```python
from build123d import *

# Parameters (mm, degrees)
SKETCH1_W                                            = 130
SKETCH1_H                                            = 10
BOSS_EXTRUDE1_DEPTH                                  = 10
CBORE_FOR_M3_HEXAGON_SOCKET_HEAD_CAP_SCR_D           = 3.2
CBORE_FOR_M3_HEXAGON_SOCKET_HEAD_CAP_SCR_CBORE_D     = 6
CBORE_FOR_M3_HEXAGON_SOCKET_HEAD_CAP_SCR_CBORE_DEPTH = 3.4
BOSS_EXTRUDE2_DEPTH                                  = 130


with BuildPart() as part:
    # Sketch1 → Boss-Extrude1 (new body)
    with BuildSketch(Plane.XY):
        with Locations((0, 5)):
            Rectangle(SKETCH1_W, SKETCH1_H)
    extrude(amount=BOSS_EXTRUDE1_DEPTH)

    # CBORE for M3 Hexagon socket head cap screws1 (through all)
    with Locations(Plane.XY.offset(10)):
        with Locations((-60, 5), (0, 5), (60, 5)):
            CounterBoreHole(CBORE_FOR_M3_HEXAGON_SOCKET_HEAD_CAP_SCR_D / 2, CBORE_FOR_M3_HEXAGON_SOCKET_HEAD_CAP_SCR_CBORE_D / 2, CBORE_FOR_M3_HEXAGON_SOCKET_HEAD_CAP_SCR_CBORE_DEPTH)

    # Sketch4 → Boss-Extrude2 (add)
    with BuildSketch(Plane.ZY.offset(65)):
        Polygon((10, 10), (0, 10), (0, 20), align=None)
    extrude(amount=-BOSS_EXTRUDE2_DEPTH)


solid = part.part
```
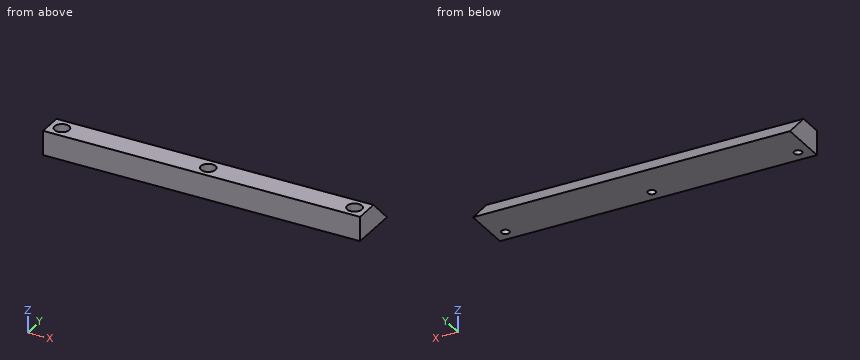
For this review, take the finished solid that the model builds, in its own axes (mm). Round coordinates to 2 decimals unless told otherwise and drop trailing zeros. Loops run counter-clockwise (first coordinate to the right, second up) from the corner with the lowest first, then second, coordinate; pieces in that order, holes last.
Q1. Add section D-D on y = 14.25. Write out the cut boundary in (x, z).
Result sheet:
outline: (-65, 0) - (65, 0) - (65, 5.75) - (-65, 5.75) - close
Q2. Add section A-A on y = 5. Write out the cut boundary in (x, z), plus the area to 3 significant figures.
Result sheet:
outline: (-65, 0) - (-61.6, 0) - (-61.6, 6.6) - (-63, 6.6) - (-63, 10) - (-65, 10) - close; (-58.4, 0) - (-1.6, 0) - (-1.6, 6.6) - (-3, 6.6) - (-3, 10) - (-57, 10) - (-57, 6.6) - (-58.4, 6.6) - close; (1.6, 0) - (58.4, 0) - (58.4, 6.6) - (57, 6.6) - (57, 10) - (3, 10) - (3, 6.6) - (1.6, 6.6) - close; (61.6, 0) - (65, 0) - (65, 10) - (63, 10) - (63, 6.6) - (61.6, 6.6) - close
area: 1,180 mm2
Q3. Insertion check: pin 1 Ø3.5 at (x, y) = (-60, 5) entering from +Z; pin 2 Ø3 at (x, y) = (0, 5) entering from +Z; pin 3 Ø1.5 at (x, y) = (48, 18) entering from +Z. Each pin has a flat end and moves straight along its axis. Give the tip position at first contact, or say it passes through.
Result sheet:
pin 1: stops at z = 6.6
pin 2: passes through
pin 3: stops at z = 2.75
Q4. Add section C-C on x = 60. Write out the cut boundary in (y, z), plus the area to 3 significant figures.
Result sheet:
outline: (0, 0) - (3.4, 0) - (3.4, 6.6) - (2, 6.6) - (2, 10) - (0, 10) - close; (6.6, 0) - (20, 0) - (10, 10) - (8, 10) - (8, 6.6) - (6.6, 6.6) - close
area: 108 mm2
Q5. Add section B-B on z = 8.5. Write out the cut boundary in (x, y).
Result sheet:
outline: (-65, 0) - (65, 0) - (65, 11.5) - (-65, 11.5) - close; hole circle Ø6 at (-60, 5); hole circle Ø6 at (0, 5); hole circle Ø6 at (60, 5)
Q6. To check wall thickness, follow line 1 along X through (y, z) = (6, 9); line 2 along Y through (x, z) = (60, 4.75); line 3 along Y through (x, z) = (-60, 3). State the ranges of each line that lie inside material, in increasing order.
Result sheet:
line 1: x = -65 to -62.83, -57.17 to -2.83, 2.83 to 57.17, 62.83 to 65
line 2: y = 0 to 3.4, 6.6 to 15.25
line 3: y = 0 to 3.4, 6.6 to 17
